from build123d import *

# Parameters (mm, degrees)
PAD078_DEPTH            = 1.6
PAD079_DEPTH            = 1.6
LINEARPATTERN001_COUNT  = 2
LINEARPATTERN001_PITCH  = 8.4
FILLET004_R             = 1
FILLET005_R             = 1
FILLET006_R             = 1
FILLET007_R             = 1.5
BODY025_PLACEMENT_ANGLE = 90


with BuildPart() as part:
    # Sketch108 → Pad078 (new body)
    with BuildSketch(Plane.XY):
        with BuildLine():
            Line((-4.5, 5), (4.5, 5))
            Line((4.5, 5), (4.5, 1.2))
            Line((0, 1.2), (4.5, 1.2))
            ThreePointArc((0, 1.2), (-1.2, 0), (0, -1.2))
            Line((4.5, -1.2), (0, -1.2))
            Line((4.5, -1.2), (4.5, -5))
            Line((4.5, -5), (-4.5, -5))
            Line((-4.5, -5), (-4.5, 5))
        make_face()
    extrude(amount=PAD078_DEPTH)

    # Sketch109 (on DatumPlane) → Pad079 (join)
    with BuildSketch(Plane.XZ.offset(5)):
        Polygon((-4.5, 0), (-4.5, -6), (-2.5, -6), (-2.5, -4.4), (0.5, 0), align=None)
    pad079 = extrude(amount=-PAD079_DEPTH)

    # LinearPattern001: Pad079 ×2
    with Locations(*[(0, i * LINEARPATTERN001_PITCH, 0) for i in range(1, LINEARPATTERN001_COUNT)]):
        add(pad079)

    # Fillet004
    fillet004_edges = [part.edges().sort_by_distance(p)[0] for p in [
        (-2.5, -4.2, -6),
        (-2.5, 4.2, -6),
    ]]
    fillet(fillet004_edges, radius=FILLET004_R)

    # Fillet005
    fillet005_edges = [part.edges().sort_by_distance(p)[0] for p in [
        (-2.5, -4.2, -4.4),
        (-2.5, 4.2, -4.4),
    ]]
    fillet(fillet005_edges, radius=FILLET005_R)

    # Fillet006
    fillet006_edges = [part.edges().sort_by_distance(p)[0] for p in [
        (4.5, -5, 0.8),
        (4.5, 5, 0.8),
    ]]
    fillet(fillet006_edges, radius=FILLET006_R)

    # Fillet007
    fillet007_edges = [part.edges().sort_by_distance(p)[0] for p in [
        (4.5, -1.2, 0.8),
        (4.5, 1.2, 0.8),
    ]]
    fillet(fillet007_edges, radius=FILLET007_R)


with BuildPart() as part_1:
    # Body025 placement: moved
    add(part.part.moved(Location((22.4, 32.5, 16.4))).rotate(Axis((22.4, 32.5, 16.4), (0, 0, 1)), BODY025_PLACEMENT_ANGLE))


solid = part_1.part
Geometry: final body of the model. Coordinates: model frame, mm. A direction names the side the tool comes from. Give positions to 0.01 mm unless a question says otherwise; leave off trailing zeros. Order: outer loops, then holes, each group sorted by start corner. A loop starts at its lowest first (then second) coordinate and runs counter-clockwise, first axis right, second up. Notation, with made-up numbers: (-20.75, 30.25) -> (-9.75, 30.25) arc R32 ccw to (-9.75, 60.25) -> close; hole circle Ø6 at (72, -40). An arc over 180 degrees is marked (long way). Answer as a JSON object with one key per item and string values.
Q1. Draft query along X for faces 4 (the flat face through (19, 30, 14)), 5 (the flat face through (27.4, 31, 15)), 6 (the flat face through (19, 37, 17)). Return one class per face: released by +X, released by -X, zero draft, split by the parting line, or undercut.
Entries:
{"face 4": "undercut", "face 5": "released by +X", "face 6": "zero draft"}
Q2. Access query for faces 1 (the flat face through (25.8, 30, 14)), 2 (the cylindrical face through (20.77, 36.55, 17.21)), 3 (the flat face through (26.61, 31.57, 14.3)). Directions: +Z, -Z, +X, -X, +Y, -Y. A direction counts if a zero-diameter tool reaches every point of the face in a straight line with its end or side. Return the directions, or none.
Entries:
{"face 1": "-Z, +Y, -Y", "face 2": "+Z, -Z, +Y", "face 3": "-Z, +X, -X, +Y"}
Q3. Section B-B (z = 13.5). Output: boundary loops of the cut face in (x, y), plus the area to 3 significant figures.
Entries:
{"outline": "(17.4, 28) -> (19, 28) -> (19, 31.02) -> (17.4, 31.02) -> close; (25.8, 28) -> (27.4, 28) -> (27.4, 31.02) -> (25.8, 31.02) -> close", "area": "9.67 mm^2"}
Q4. Section C-C (x = 18.75). Output: boundary loops of the cut face in (y, z), plus the area to 3 significant figures.
Entries:
{"outline": "(28, 10.4) -> (29, 10.4) arc R1 ccw to (30, 11.4) -> (30, 11.69) arc R1 cw to (30.17, 12.25) -> (33, 16.4) -> (37, 16.4) -> (37, 18) -> (28, 18) -> close", "area": "32.8 mm^2"}
Q5. Section A-A (y = 34.75). Output: boundary loops of the cut face in (x, z).
Entries:
{"outline": "(17.4, 16.4) -> (21.2, 16.4) -> (21.2, 18) -> (17.4, 18) -> close; (23.6, 16.4) -> (27.4, 16.4) -> (27.4, 18) -> (23.6, 18) -> close"}
Q6. Material intervals for probe 1 along X at (y, z) = (29.25, 13.5); probe 2 along Z at (x, y) = (22.25, 29.5); probe 3 along X at (y, z) = (31.5, 17.25), sorted ascending.
Entries:
{"probe 1": "x = 17.4 to 19, 25.8 to 27.4", "probe 2": "z = 16.4 to 18", "probe 3": "x = 17.4 to 21.74, 23.06 to 27.4"}
Q7. First-contact query: pin 1 (3 mm diameter, centred on x = 22.5, z = 12, fed in from -Y). Flat tip, straight axial feed; report the tip coordinate or a pass-through.
Entries:
{"pin 1": "passes through"}
Q8. Section D-D (y = 28.75). Output: boundary loops of the cut face in (x, z), plus the area to 3 significant figures.
Entries:
{"outline": "(17.4, 10.4) -> (19, 10.4) -> (19, 16.4) -> (25.8, 16.4) -> (25.8, 10.4) -> (27.4, 10.4) -> (27.4, 18) -> (17.4, 18) -> close", "area": "35.2 mm^2"}
